Design review of the part shown in the three views and the two pictorial views. Dimensions are in mm from the part's minimum x, y and z. A direction names the side the tool comes from. Round coordinates to 2 decimals unless told otherwise and drop trailing zeros. Loops run counter-clockwise (first coordinate to the right, second up) from the corner with the lowest first, then second, coordinate; pieces in that order, holes last. Notation, with made-up numbers: (11.5, 89) -> (20.5, 89) arc R25 ccw to (20.5, 113) -> close; hole circle Ø10 at (80, 14.5). An arc over 180 degrees is marked (long way). One line per question, with ' | ' between items. Start each with the question number.
1. For the marked faces 1, 2 and 3, list the 3-axis set-ups (+Z, -Z, +X, -X, +Y, -Y) from which the entire face can be reached by the end or side of a thin tool; tool diameter is ignored.
2. Consider section D-D (y = 19). Write out the cut boundary in (x, z), and give its area (3 significant figures).
3. Consider section B-B (y = 4.5). Write out the cut boundary in (x, z), and give its area (3 significant figures).
4. Wall thickness on line 1 along X through (y, z) = (6, 7.75); line 2 along Y through (x, z) = (31.5, 0.5); line 3 along Z through (x, y) = (36, 15): over which ranges is each line inside the solid? List them lowest first.
5. For pin 1 Ø3.5 at (y, z) = (7, 5) entering from -X; pin 2 Ø2 at (x, z) = (26, 4) entering from +Y; pin 3 Ø12.5 at (x, y) = (30.5, 19.5) entering from +Z, all flat-tipped, find the tip position at first contact; note any pin that passes through.
6. Consider section A-A (z = 3.5). Write out the cut boundary in (x, y).
7. Consider section C-C (x = 16.5). Write out the cut boundary in (y, z), and give its area (3 significant figures).
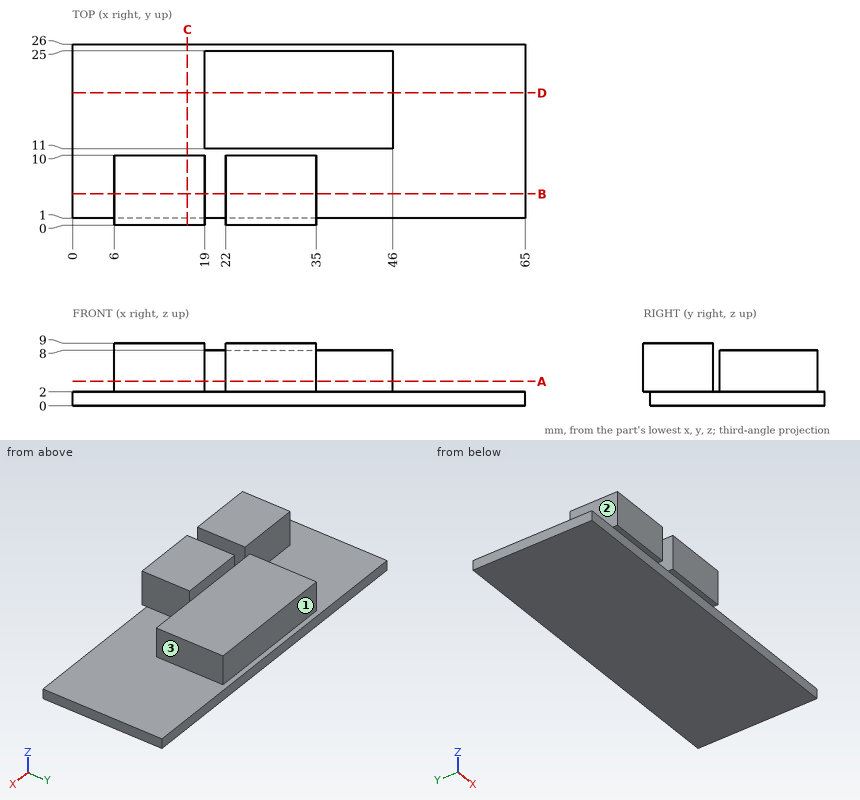
Answer block:
1) face 1: +Z, +X, -X, +Y | face 2: +Z, -X, +Y, -Y | face 3: +Z, +X, +Y, -Y
2) outline: (0, 0) -> (65, 0) -> (65, 2) -> (46, 2) -> (46, 8) -> (19, 8) -> (19, 2) -> (0, 2) -> close | area: 292 mm2
3) outline: (0, 0) -> (65, 0) -> (65, 2) -> (35, 2) -> (35, 9) -> (22, 9) -> (22, 2) -> (19, 2) -> (19, 9) -> (6, 9) -> (6, 2) -> (0, 2) -> close | area: 312 mm2
4) line 1: x = 6 to 19, 22 to 35 | line 2: y = 1 to 26 | line 3: z = 0 to 8
5) pin 1: stops at x = 6 | pin 2: stops at y = 25 | pin 3: stops at z = 8
6) outline: (6, 0) -> (19, 0) -> (19, 10) -> (6, 10) -> close; (19, 11) -> (46, 11) -> (46, 25) -> (19, 25) -> close; (22, 0) -> (35, 0) -> (35, 10) -> (22, 10) -> close
7) outline: (0, 2) -> (1, 2) -> (1, 0) -> (26, 0) -> (26, 2) -> (10, 2) -> (10, 9) -> (0, 9) -> close | area: 120 mm2
